The listing builds one solid part. Answer for the finished solid, in the listing's coordinates (mm). A direction names the side the tool comes from. Coordinates: 2 decimals unless noted, no trailing zeros. Order: outer loops, then holes, each group sorted by start corner. A loop starts at its lowest first (then second) coordinate and runs counter-clockwise, first axis right, second up. Notation, with made-up numbers: (-20, -2) -> (-1, -2) arc R24 cw to (-1, 15) -> close; hole circle Ø8 at (-11, -32.75). An arc over 180 degrees is marked (long way). Return JSON: item names as keys, results as strings.
from build123d import *

# Parameters (mm, degrees)
BASE_EXTRUDE_DEPTH  = 5.08
SHELL1_T            = -1.524
SKETCH2_R           = 2.0955
CUT_EXTRUDE1_DEPTH  = 17.756782537
SKETCH4_R           = 5.08
BOSS_EXTRUDE1_DEPTH = 7.366
SKETCH5_R           = 2.794
CUT_EXTRUDE2_DEPTH  = 21.955
SKETCH3_R           = 3.556
CUT_EXTRUDE3_DEPTH  = 2.159
SKETCH6_R           = 3.937
CUT_EXTRUDE4_DEPTH  = 2.159
FILLET1_R           = 1.016


with BuildPart() as part:
    # Sketch1 → Base-Extrude (new, symmetric)
    with BuildSketch(Plane.XY):
        with BuildLine():
            Line((-5.08, 0), (5.08, 0))
            Line((5.08, 0), (5.08, 7.239))
            ThreePointArc((5.08, 7.239), (0, 12.319), (-5.08, 7.239))
            Line((-5.08, 7.239), (-5.08, 0))
        make_face()
    extrude(amount=BASE_EXTRUDE_DEPTH, both=True)

    # Shell1
    shell1_openings = [part.faces().sort_by_distance(p)[0] for p in [
        (5.08, 3.6195, 0),
        (0, 12.319, 0),
        (-5.08, 3.6195, 0),
    ]]
    offset(amount=SHELL1_T, openings=shell1_openings, kind=Kind.INTERSECTION)

    # Sketch2 → Cut-Extrude1 (cut, through all)
    with BuildSketch(Plane.XY.offset(5.08)):
        with Locations((0, 7.239)):
            Circle(SKETCH2_R)
    extrude(amount=-CUT_EXTRUDE1_DEPTH, mode=Mode.SUBTRACT)

    # Sketch4 → Boss-Extrude1 (add)
    with BuildSketch(Plane.XZ):
        Circle(SKETCH4_R)
    extrude(amount=BOSS_EXTRUDE1_DEPTH)

    # Sketch5 → Cut-Extrude2 (cut, through all)
    with BuildSketch(Plane.XZ.offset(7.366)):
        Circle(SKETCH5_R)
    extrude(amount=-CUT_EXTRUDE2_DEPTH, mode=Mode.SUBTRACT)

    # Sketch3 → Cut-Extrude3 (cut)
    with BuildSketch(Plane(origin=(0, 1.524, 0), x_dir=(-1, 0, 0), z_dir=(0, 1, 0))):
        Circle(SKETCH3_R)
    extrude(amount=-CUT_EXTRUDE3_DEPTH, mode=Mode.SUBTRACT)

    # Sketch6 → Cut-Extrude4 (cut)
    with BuildSketch(Plane.XZ.offset(7.366)):
        Circle(SKETCH6_R)
    extrude(amount=-CUT_EXTRUDE4_DEPTH, mode=Mode.SUBTRACT)

    # Fillet1
    fillet1_edges = [part.edges().sort_by_distance(p)[0] for p in [
        (-5.08, -7.366, 0),
    ]]
    fillet(fillet1_edges, radius=FILLET1_R)


solid = part.part
1. Consider line 1 (Z direction, x = 0, y = 0.1); line 2 (Z direction, x = 0, y = -5.7). Determine where each line is inside the solid, lowest interval first. Write a range as from..to.
Answer block:
{"line 1": "z = -5.08..-3.56, 3.56..5.08", "line 2": "z = -5.08..-3.94, 3.94..5.08"}
2. Determine the mould class of faces 4 (the face through (-0.454, 5.193, 4.329)), 5 (the face through (-0.1, 4.9, 5.08)), 6 (the face through (5.08, 1, 0)) for opening direction X: pulls with the +X half, pulls with the -X half, needs draft (parallel to the pull), parting line crosses it, or undercut.
Answer block:
{"face 4": "undercut", "face 5": "needs draft", "face 6": "pulls with the +X half"}
3. For faces 1 (the face through (4, 0, -4)), 2 (the face through (3, -0.635, -1)), 3 (the face through (-0.1, 4.6, -3.556)), determine the directions among +Z, -Z, +X, -X, +Y, -Y from which every point of the face is accessible in a straight line to the end or side of a thin tool.
Answer block:
{"face 1": "-Z, +X, -Y", "face 2": "+Y", "face 3": "+X, -X, +Y"}
4. The part is cut by section A-A on y = 10. Give the vertices of the cut face in (x, z).
Answer block:
{"outline": "(-4.26, -5.08) -> (4.26, -5.08) -> (4.26, -3.56) -> (-4.26, -3.56) -> close; (-4.26, 3.56) -> (4.26, 3.56) -> (4.26, 5.08) -> (-4.26, 5.08) -> close"}
5. The part is cut by section C-C on y = -5.5. Give the vertices of the cut face in (x, z).
Answer block:
{"outline": "circle Ø10.16 at (0, 0); hole circle Ø7.87 at (0, 0)"}
6. The part is cut by section B-B on x = -0.5. Give the number of separate pieces and of enclosed holes in the cut face, and give its area (3 significant figures).
Answer block:
{"separate pieces": "4", "enclosed holes": "0", "area": "52.7 mm2"}
7. Each of these flat-tipped pins is pushed along its axis until it touches: pin 1 Ø6 at (x, z) = (2, 0) entering from -Y; pin 2 Ø5.5 at (x, z) = (3.5, -1.5) entering from +Y; pin 3 Ø3 at (x, z) = (0, 2) entering from -Y; pin 4 Ø4 at (x, z) = (-2.5, -4) entering from +Y. Where does it stop, or does it pass through?
Answer block:
{"pin 1": "stops at y = -7.37", "pin 2": "stops at y = 12.04", "pin 3": "stops at y = -5.21", "pin 4": "stops at y = 12.29"}
